Here's how the part is built. I have some questions about the finished solid (model axes, mm). Coordinates: 2 decimals unless noted, no trailing zeros. Loops run counter-clockwise (first coordinate to the right, second up) from the corner with the lowest first, then second, coordinate; pieces in that order, holes last.
```python
from build123d import *

# Parameters (mm, degrees)
BOSS_EXTRUDE1_DEPTH = 5
SKETCH4_R           = 2.0701
CUT_EXTRUDE1_DEPTH  = 712.6709914
LPATTERN2_COUNT     = 24
LPATTERN2_PITCH     = 25.4
LPATTERN3_COUNT     = 32
LPATTERN3_PITCH     = 25.4
LPATTERN4_OUTLINE_R = 2.0701
LPATTERN4_DEPTH     = 5
LPATTERN5_OUTLINE_R = 2.0701
LPATTERN5_DEPTH     = 5
FILLET1_R           = 6.35
SKETCH6_R           = 3.175
CUT_EXTRUDE2_DEPTH  = 712.6709914
LPATTERN6_COUNT     = 7
LPATTERN6_PITCH     = 40.64


# Read off the part's stored shape, not the designer's step: LPattern4, LPattern5
with BuildPart() as part:
    # Sketch1 → Boss-Extrude1 (new body)
    with BuildSketch(Plane.XY):
        Polygon((-549.275, -355.6), (-584.2, -355.6), (-584.2, -406.4), (25.4, -406.4), (25.4, -355.6), (-9.525, -355.6), (-9.525, -254), (25.4, -254), (25.4, -68.43150672), (-100.0125, -68.43150672), (-100.0125, 68.43150672), (25.4, 68.43150672), (25.4, 254), (-9.525, 254), (-9.525, 355.6), (25.4, 355.6), (25.4, 406.4), (-79.375, 406.4), (-79.375, 254), (-479.425, 254), (-479.425, 406.4), (-584.2, 406.4), (-584.2, 355.6), (-549.275, 355.6), (-549.275, 254), (-584.2, 254), (-584.2, 68.43150672), (-458.7875, 68.43150672), (-458.7875, -68.43150672), (-584.2, -68.43150672), (-584.2, -254), (-549.275, -254), align=None)
    extrude(amount=BOSS_EXTRUDE1_DEPTH)

    # Sketch4 → Cut-Extrude1 (cut, symmetric)
    with BuildSketch(Plane.XY.offset(5)):
        with Locations((-571.5, 393.7)):
            Circle(SKETCH4_R)
    cut_extrude1 = extrude(amount=CUT_EXTRUDE1_DEPTH, both=True, mode=Mode.SUBTRACT)

    # LPattern2: Cut-Extrude1 ×24, 16 skipped
    with Locations(*[(i * LPATTERN2_PITCH, 0, 0) for i in range(1, LPATTERN2_COUNT) if i not in (4, 5, 6, 7, 8, 9, 10, 11, 12, 13, 14, 15, 16, 17, 18, 19)]):
        add(cut_extrude1, mode=Mode.SUBTRACT)

    # LPattern3: Cut-Extrude1 ×32, 13 skipped
    with Locations(*[(0, -i * LPATTERN3_PITCH, 0) for i in range(1, LPATTERN3_COUNT) if i not in (2, 3, 4, 5, 14, 15, 16, 17, 18, 26, 27, 28, 29)]):
        add(cut_extrude1, mode=Mode.SUBTRACT)

    # LPattern4 outline → LPattern4 (cut)
    with BuildSketch(Plane.XY):
        with Locations((12.7, -393.7)):
            Circle(LPATTERN4_OUTLINE_R)
        with Locations((-12.7, -393.7)):
            Circle(LPATTERN4_OUTLINE_R)
        with Locations((-38.1, -393.7)):
            Circle(LPATTERN4_OUTLINE_R)
        with Locations((-63.5, -393.7)):
            Circle(LPATTERN4_OUTLINE_R)
        with Locations((-88.9, -393.7)):
            Circle(LPATTERN4_OUTLINE_R)
        with Locations((-114.3, -393.7)):
            Circle(LPATTERN4_OUTLINE_R)
        with Locations((-139.7, -393.7)):
            Circle(LPATTERN4_OUTLINE_R)
        with Locations((-165.1, -393.7)):
            Circle(LPATTERN4_OUTLINE_R)
        with Locations((-190.5, -393.7)):
            Circle(LPATTERN4_OUTLINE_R)
        with Locations((-215.9, -393.7)):
            Circle(LPATTERN4_OUTLINE_R)
        with Locations((-241.3, -393.7)):
            Circle(LPATTERN4_OUTLINE_R)
        with Locations((-266.7, -393.7)):
            Circle(LPATTERN4_OUTLINE_R)
        with Locations((-292.1, -393.7)):
            Circle(LPATTERN4_OUTLINE_R)
        with Locations((-317.5, -393.7)):
            Circle(LPATTERN4_OUTLINE_R)
        with Locations((-342.9, -393.7)):
            Circle(LPATTERN4_OUTLINE_R)
        with Locations((-368.3, -393.7)):
            Circle(LPATTERN4_OUTLINE_R)
        with Locations((-393.7, -393.7)):
            Circle(LPATTERN4_OUTLINE_R)
        with Locations((-419.1, -393.7)):
            Circle(LPATTERN4_OUTLINE_R)
        with Locations((-444.5, -393.7)):
            Circle(LPATTERN4_OUTLINE_R)
        with Locations((-469.9, -393.7)):
            Circle(LPATTERN4_OUTLINE_R)
        with Locations((-495.3, -393.7)):
            Circle(LPATTERN4_OUTLINE_R)
        with Locations((-520.7, -393.7)):
            Circle(LPATTERN4_OUTLINE_R)
        with Locations((-546.1, -393.7)):
            Circle(LPATTERN4_OUTLINE_R)
    extrude(amount=LPATTERN4_DEPTH, mode=Mode.SUBTRACT)

    # LPattern5 outline → LPattern5 (cut)
    with BuildSketch(Plane.XY):
        with Locations((12.7, -368.3)):
            Circle(LPATTERN5_OUTLINE_R)
        with Locations((12.7, -241.3)):
            Circle(LPATTERN5_OUTLINE_R)
        with Locations((12.7, -215.9)):
            Circle(LPATTERN5_OUTLINE_R)
        with Locations((12.7, -190.5)):
            Circle(LPATTERN5_OUTLINE_R)
        with Locations((12.7, -165.1)):
            Circle(LPATTERN5_OUTLINE_R)
        with Locations((12.7, -139.7)):
            Circle(LPATTERN5_OUTLINE_R)
        with Locations((12.7, -114.3)):
            Circle(LPATTERN5_OUTLINE_R)
        with Locations((12.7, -88.9)):
            Circle(LPATTERN5_OUTLINE_R)
        with Locations((12.7, 88.9)):
            Circle(LPATTERN5_OUTLINE_R)
        with Locations((12.7, 114.3)):
            Circle(LPATTERN5_OUTLINE_R)
        with Locations((12.7, 139.7)):
            Circle(LPATTERN5_OUTLINE_R)
        with Locations((12.7, 165.1)):
            Circle(LPATTERN5_OUTLINE_R)
        with Locations((12.7, 190.5)):
            Circle(LPATTERN5_OUTLINE_R)
        with Locations((12.7, 215.9)):
            Circle(LPATTERN5_OUTLINE_R)
        with Locations((12.7, 241.3)):
            Circle(LPATTERN5_OUTLINE_R)
        with Locations((12.7, 368.3)):
            Circle(LPATTERN5_OUTLINE_R)
    extrude(amount=LPATTERN5_DEPTH, mode=Mode.SUBTRACT)

    # Fillet1
    fillet1_edges = [part.edges().sort_by_distance(p)[0] for p in [
        (-549.275, -355.6, 2.5),
        (-549.275, -254, 2.5),
        (-458.7875, -68.43150672, 2.5),
        (-458.7875, 68.43150672, 2.5),
        (-549.275, 254, 2.5),
        (-549.275, 355.6, 2.5),
        (-479.425, 254, 2.5),
        (-79.375, 254, 2.5),
        (-9.525, 355.6, 2.5),
        (-9.525, 254, 2.5),
        (-100.0125, 68.43150672, 2.5),
        (-100.0125, -68.43150672, 2.5),
        (-9.525, -254, 2.5),
        (-9.525, -355.6, 2.5),
    ]]
    fillet(fillet1_edges, radius=FILLET1_R)

    # Sketch6 → Cut-Extrude2 (cut, through all)
    with BuildSketch(Plane(origin=(0, 0, 0), x_dir=(-1, 0, 0), z_dir=(0, 0, -1))):
        with Locations((436.9527202, -330.835)):
            Circle(SKETCH6_R)
        with Locations((436.9527202, -371.475)):
            Circle(SKETCH6_R)
        with Locations((485.7877, -371.475)):
            Circle(SKETCH6_R)
        with Locations((485.7877, -330.835)):
            Circle(SKETCH6_R)
        with BuildLine():
            ThreePointArc((436.9654202, -351.155), (436.961700456, -351.146019744), (436.9527202, -351.1423))
            Line((436.9527202, -351.1423), (436.9527202, -351.1677))
            ThreePointArc((436.9527202, -351.1677), (436.961700456, -351.163980256), (436.9654202, -351.155))
        make_face()
        with BuildLine():
            Line((436.9527202, -351.1677), (436.9527202, -351.1423))
            ThreePointArc((436.9527202, -351.1423), (436.9400202, -351.155), (436.9527202, -351.1677))
        make_face()
    cut_extrude2 = extrude(amount=-CUT_EXTRUDE2_DEPTH, mode=Mode.SUBTRACT)

    # LPattern6: Cut-Extrude2 ×7
    with Locations(*[(0, i * LPATTERN6_PITCH, 0) for i in range(1, LPATTERN6_COUNT)]):
        add(cut_extrude2, mode=Mode.SUBTRACT)


solid = part.part
```
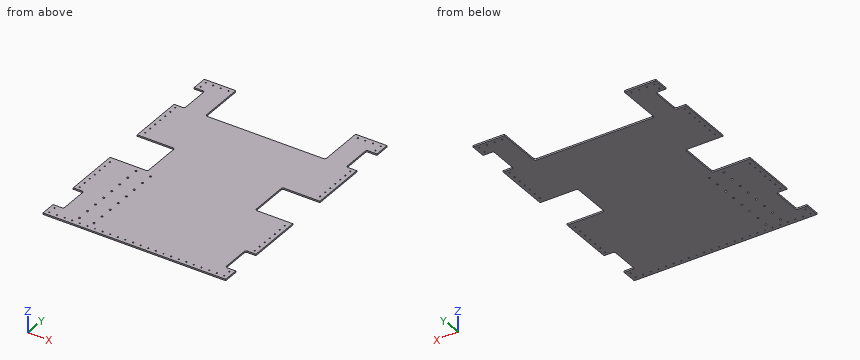
1. I need wall thicknesses on line 1 along Y through (x, z) = (-0.5, 3.45); line 2 along Y through (x, z) = (-140.5, 1.35); line 3 along Y through (x, z) = (-21, 2.8). Which ranges of each line are inside material? Lowest first, please.
2. I want a section at A-A (x = -253). Please give me the cut outline in (y, z).
3. I want a section at B-B (y = 7). Please give me the cut outline in (x, z).
4. For pin 1 (1.5 mm diameter, centred on x = -300, z = 3, fed in from +Y); pin 2 (1 mm diameter, centred on y = -26.5, z = 3, fed in from -X); pin 3 (3 mm diameter, centred on y = -287.5, z = 4, fed in from +X) (3 decimals), each with a flat end and sliding along its axis, tell me the tip position at first contact or that it passes through.
Response values:
1. line 1: y = -406.4 to -355.6, -254 to -68.43, 68.43 to 254, 355.6 to 406.4
1. line 2: y = -406.4 to -395.61, -391.79 to 254
1. line 3: y = -406.4 to -68.43, 68.43 to 406.4
2. outline: (-406.4, 0) - (254, 0) - (254, 5) - (-406.4, 5) - close
3. outline: (-458.79, 0) - (-100.01, 0) - (-100.01, 5) - (-458.79, 5) - close
4. pin 1: stops at y = 254
4. pin 2: stops at x = -458.79
4. pin 3: stops at x = -9.525
